Autodesk Inventor part; units mm, degrees
ref_plane "YZ Plane" through (0, 0, 0) normal (1, 0, 0) x (0, 1, 0)
ref_plane "XZ Plane" through (0, 0, 0) normal (0, 1, 0) x (-1, 0, 0)
ref_plane "XY Plane" through (0, 0, 0) normal (0, 0, 1) x (1, 0, 0)
sketch "Sketch3" plane through (0, 0, 0) normal (0, 0, 1) x (1, 0, 0)
  circle A0 centre (0, 0) radius 4.45
  dimension "d11" = 8.9
extrude "Extrusion3" add sketch "Sketch3" along normal blind 6
sketch "Sketch4" plane through (0, 0, 6) normal (0, 0, 1) x (1, 0, 0)
  circle A0 centre (0, 0) radius 30
  dimension "d14" = 60
extrude "Extrusion4" add sketch "Sketch4" along normal blind 8
ref_plane "Work Plane2" through (0, 0, 8) normal (0, 0, 1) x (1, 0, 0)
ref_plane "Work Plane1" through (0, 0, 10) normal (0, 0, 1) x (1, 0, 0)
sketch "Sketch5" plane through (0, 0, 8) normal (0, 0, 1) x (1, 0, 0)
  circle A0 centre (0, 0) radius 28.5
  circle A1 centre (0, 0) radius 30
  dimension "d17" = 57
  dimension "d18" = 60
extrude "Extrusion5" cut sketch "Sketch5" along normal mid plane 2
mirror "Mirror1" about plane through (0, 0, 10) normal (0, 0, 1) of "Extrusion5"
sketch "Sketch7" plane through (0, 0, 0) normal (0, 0, -1) x (-1, 0, 0)
  line L0 (-3.4063, 0) -> (1.7033, -2.95)
  line L1 (1.7033, -2.95) -> (1.7033, 2.95)
  line L2 (-3.4063, 0) -> (1.7033, 2.95)
  dimension "d29" = 5.9
  dimension "d30" = 5.9
  dimension "d34" = 5.9
extrude "Extrusion7" add sketch "Sketch7" along normal blind 12
sketch "Sketch8" plane through (-1.7033, -2.95, 0) normal (-1, 0, 0) x (0, 0, 1)
  line L0 (0, 2.95) -> (-12, 2.95)
  circle A0 centre (-10.9447, 2.95) radius 0.75
  dimension "d37" = 1.5
extrude "Extrusion8" cut sketch "Sketch8" against normal blind 12
ref_plane "Work Plane3" through (0, 0, 10) normal (0, 0, 1) x (1, 0, 0)
ref_plane "Work Plane4" through (0, 0, 12) normal (0, 0, 1) x (1, 0, 0)
equation "\"d29\" = d34"
equation "\"d30\" = d34"
properties part number "PulleyAdapter"
Verification items for the finished model (mm, model axes). A direction names the side the tool comes from. Give positions to 0.01 mm unless a question says otherwise; leave off trailing zeros. Order: outer loops, then holes, each group sorted by start corner. A loop starts at its lowest first (then second) coordinate and runs counter-clockwise, first axis right, second up. Notation, with made-up numbers: M 39,55.5 L 80,55.5 A27 cw 80,77.5 Z; hole C 73,54.25 d1. An arc over 180 degrees is marked long. Answer as a JSON object with one key per item and string values. Group by question number.
1) Cross-section at C-C (y = 1.5). Enter the section's corners in (x, z).
2) Mould release check, pull along Z, two halves, no side actions. Record for faces 6 (the face through (-11, -27, 13)), 7 (the face through (0, 0, -12)), 8 (the face through (11, -27, 7)), 9 (the face through (-29.97, -1.32, 9.99)): released by +Z, released by -Z, zero draft, split by the parting line, or undercut.
3) Access from +Z, -Z, +X, -X, +Y, -Y to the whole of each face (thin tool, end or side, straight path). Record for faces 1 (the face through (26.327, -10.916, 12.014)), 2 (the face through (0.887, -1.454, -5.916)), 3 (the face through (0.887, 1.454, -5.916)), 4 (the face through (-0.965, 4.344, 2.958)), 5 (the face through (-1.703, 0, -6)).
4) Scan lines: line 1 along Z through (x, y) = (0, 0); line 2 along Z through (x, y) = (7.5, 15.5); line 3 along Y through (x, z) = (-1.5, 8). Record each from-to range of solid material in increasing order. Write a range as [from, to].
5) Cross-section at B-B (z = -8.5). Enter the section's corners in (x, y), then the cut area to 3 significant figures.
6) Depth check by flat-ended pin: pin 1 Ø6 at (x, z) = (-1.5, -2) entering from +Y; pin 2 Ø4 at (y, z) = (-10.5, 10.5) entering from -X; pin 3 Ø4 at (x, z) = (-17.5, 8) entering from -Y; pin 4 Ø10 at (x, y) = (1, 1.5) entering from -Z. Enter the tip coordinate at first touch or a pass-through.
7) Cross-section at A-A (x = -21). Enter the section's corners in (y, z), then the cut area to 3 significant figures.
Result sheet:
{
 "1": {"outline": "M -29.96,6 L -4.19,6 L -4.19,0 L -1.7,0 L -1.7,-12 L 0.81,-12 L 0.81,0 L 4.19,0 L 4.19,6 L 29.96,6 L 29.96,7 L 28.46,7 L 28.46,9 L 29.96,9 L 29.96,11 L 28.46,11 L 28.46,13 L 29.96,13 L 29.96,14 L -29.96,14 L -29.96,13 L -28.46,13 L -28.46,11 L -29.96,11 L -29.96,9 L -28.46,9 L -28.46,7 L -29.96,7 Z"},
 "2": {"face 6": "undercut", "face 7": "released by -Z", "face 8": "undercut", "face 9": "zero draft"},
 "3": {"face 1": "none", "face 2": "-Z, +X, -Y", "face 3": "-Z, +X, +Y", "face 4": "-Z", "face 5": "-Z, -X, +Y, -Y"},
 "4": {"line 1": "z = [-12, -11.69], [-10.19, 14]", "line 2": "z = [6, 14]", "line 3": "y = [-28.46, 28.46]"},
 "5": {"outline": "M -1.7,-2.95 L 3.41,0 L -1.7,2.95 Z", "area": "15.1 mm2"},
 "6": {"pin 1": "stops at y = 4.45", "pin 2": "stops at x = -28.77", "pin 3": "stops at y = -25.52", "pin 4": "stops at z = -12"},
 "7": {"outline": "M -21.42,6 L 21.42,6 L 21.42,7 L 19.27,7 L 19.27,9 L 21.42,9 L 21.42,11 L 19.27,11 L 19.27,13 L 21.42,13 L 21.42,14 L -21.42,14 L -21.42,13 L -19.27,13 L -19.27,11 L -21.42,11 L -21.42,9 L -19.27,9 L -19.27,7 L -21.42,7 Z", "area": "326 mm2"}
}
